Check sheet for the drawn part. Datum: minimum x, y, z corner. Units: mm. Coordinates: 2 decimals unless noted, no trailing zeros. Loops run counter-clockwise (first coordinate to the right, second up) from the corner with the lowest first, then second, coordinate; pieces in that order, holes last. Notation, with made-up numbers: (-4.5, 11) - (41.5, 11) arc R33 ccw to (41.5, 46) - close; hole circle Ø11 at (48.5, -18). An arc over 180 degrees is marked (long way). Answer as CSV lines item,"result". Start each with the question number.
1. Material ranges on line 1 (Z direction, x = 12.7, y = 29.5) (3 decimals); line 2 (Y direction, x = 1.75, z = 48); line 3 (X direction, y = 15, z = 7), recorded low to high. Write a range as [from, to].
2. Cross-section at A-A (z = 6.35). Enter the section's corners in (x, y) (3 decimals), plus the area to 3 significant figures.
3. Gauge pin test, flat end, axial feed: P1, Ø7.5, axis at x = 9.5, z = 20.5, coming from the -Y side. Record the tip position at first contact, or that the pin passes through.
4. Cross-section at D-D (x = 7.25). Enter the section's corners in (y, z), plus the area to 3 significant figures.
5. Release check for a two-part mould opening along Z. For the marked faces 1, 2 and 3 record: pulls with the +Z half, pulls with the -Z half, needs draft (parallel to the pull), parting line crosses it, or undercut.
6. Cross-section at B-B (x = 12.7). Enter the section's corners in (y, z) (3 decimals).
7. Cross-section at C-C (z = 44.45). Enter the section's corners in (x, y) (3 decimals), plus the area to 3 significant figures.
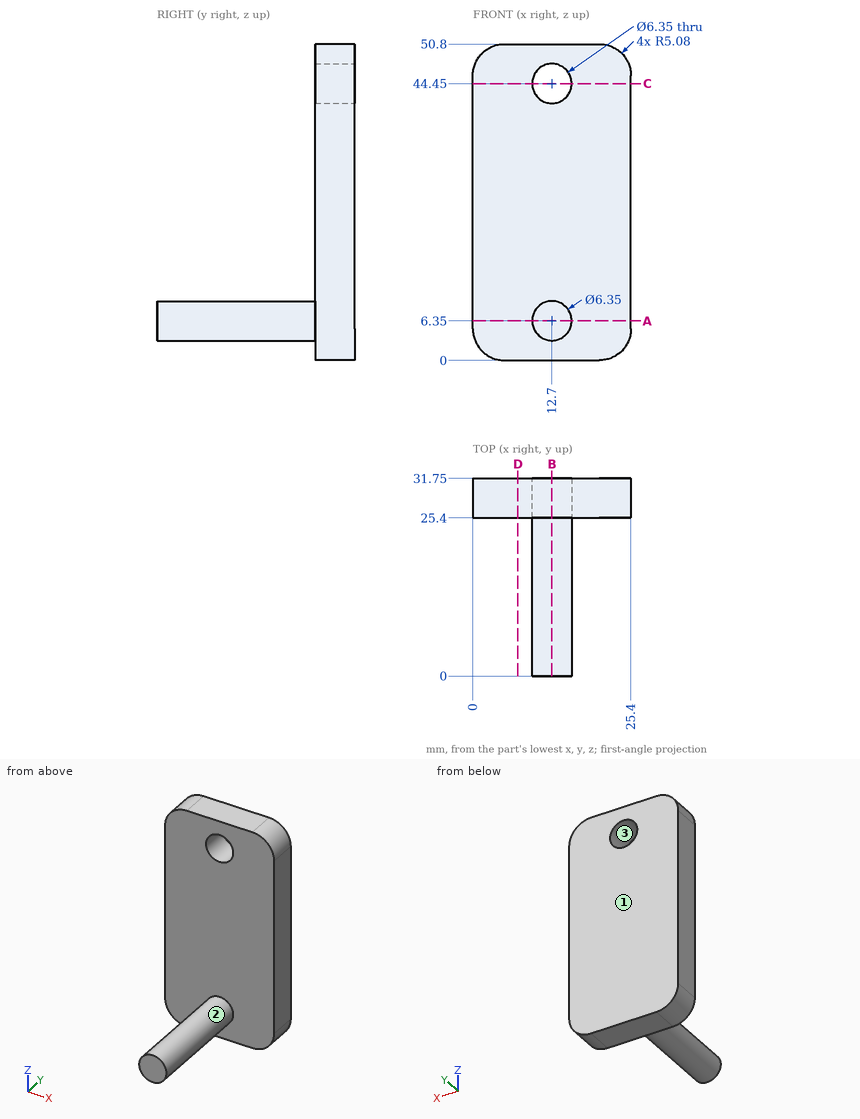
Values follow:
1,line 1,"z = [0, 41.275], [47.625, 50.8]"
1,line 2,"y = [25.4, 31.75]"
1,line 3,"x = [9.59, 15.81]"
2,outline,"(0, 25.4) - (9.525, 25.4) - (9.525, 0) - (15.875, 0) - (15.875, 25.4) - (25.4, 25.4) - (25.4, 31.75) - (0, 31.75) - close"
2,area,"323 mm²"
3,P1,"stops at y = 25.4"
4,outline,"(25.4, 0) - (31.75, 0) - (31.75, 50.8) - (25.4, 50.8) - close"
4,area,"323 mm²"
5,face 1,"needs draft"
5,face 2,"parting line crosses it"
5,face 3,"undercut"
6,outline,"(0, 3.175) - (25.4, 3.175) - (25.4, 0) - (31.75, 0) - (31.75, 41.275) - (25.4, 41.275) - (25.4, 9.525) - (0, 9.525) - close; (25.4, 47.625) - (31.75, 47.625) - (31.75, 50.8) - (25.4, 50.8) - close"
7,outline,"(0, 25.4) - (9.525, 25.4) - (9.525, 31.75) - (0, 31.75) - close; (15.875, 25.4) - (25.4, 25.4) - (25.4, 31.75) - (15.875, 31.75) - close"
7,area,"121 mm²"
